```python
from build123d import *

# Parameters (mm, degrees)
F0_W     = 50.8
F0_H     = 25.4
F0_R     = 3
F1_DEPTH = 3.5
F2_DEPTH = 10.16
F3_SIZE  = 1.27
F4_SIZE  = 3.81
F0_R_2   = 1.75
F5_DEPTH = 2.54
F6_W     = 6.391182
F6_H     = 4.83196
F7_DEPTH = 31.592


with BuildPart() as f1:
    # F0 (on Top) → F1 (new body)
    with BuildSketch(Plane.XY):
        with Locations((2.701852, 34.358082)):
            Rectangle(F0_W, F0_H)
        Polygon((-19.831223, 38.395144), (-19.831223, 44.550914), (25.234927, 44.550914), (25.234927, 38.395144), (18.497852, 38.395144), (18.497852, 30.32102), (25.234927, 30.32102), (25.234927, 24.16525), (-19.831223, 24.16525), (-19.831223, 30.32102), (-13.094148, 30.32102), (-13.094148, 38.395144), align=None, mode=Mode.SUBTRACT)
        with Locations((-16.348148, 34.358082)):
            Circle(F0_R, mode=Mode.SUBTRACT)
        with Locations((21.751852, 34.358082)):
            Circle(F0_R, mode=Mode.SUBTRACT)
    extrude(amount=F1_DEPTH)

    # F0 (on Top) → F2 (join)
    with BuildSketch(Plane.XY):
        Polygon((25.234927, 44.550914), (-19.831223, 44.550914), (-19.831223, 38.395144), (-13.094148, 38.395144), (-13.094148, 30.32102), (-19.831223, 30.32102), (-19.831223, 24.16525), (25.234927, 24.16525), (25.234927, 30.32102), (18.497852, 30.32102), (18.497852, 38.395144), (25.234927, 38.395144), align=None)
    extrude(amount=F2_DEPTH)

    # F3
    f3_edges = [f1.edges().sort_by_distance(p)[0] for p in [
        (-22.698148, 34.358082, 3.5),
        (2.701852, 21.658082, 3.5),
        (2.701852, 47.058082, 3.5),
        (28.101852, 34.358082, 3.5),
        (-22.698148, 47.058082, 1.75),
        (-22.698148, 21.658082, 1.75),
        (28.101852, 21.658082, 1.75),
        (28.101852, 47.058082, 1.75),
    ]]
    chamfer(f3_edges, length=F3_SIZE)

    # F4
    f4_edges = [f1.edges().sort_by_distance(p)[0] for p in [
        (25.234927, 41.473029, 10.16),
        (2.701852, 44.550914, 10.16),
        (25.234927, 27.243135, 10.16),
        (2.701852, 24.16525, 10.16),
        (-19.831223, 41.473029, 10.16),
        (-19.831223, 27.243135, 10.16),
    ]]
    chamfer(f4_edges, length=F4_SIZE)

    # F0 (on Top) → F5 (join)
    with BuildSketch(Plane.XY):
        with Locations((21.751852, 34.358082)):
            Circle(F0_R)
        with Locations((21.751852, 34.358082)):
            Circle(F0_R_2, mode=Mode.SUBTRACT)
        with Locations((-16.348148, 34.358082)):
            Circle(F0_R)
        with Locations((-16.348148, 34.358082)):
            Circle(F0_R_2, mode=Mode.SUBTRACT)
    extrude(amount=F5_DEPTH)

    # F6 (on face) → F7 (cut, through all)
    with BuildSketch(Plane(origin=(-13.094148, 0, 0), x_dir=(0, -1, 0), z_dir=(-1, 0, 0))):
        with Locations((-34.358082, 6.83)):
            Rectangle(F6_W, F6_H)
    extrude(amount=-F7_DEPTH, mode=Mode.SUBTRACT)


solid = f1.part
```
Here's how the part is built. I have some questions about the finished solid (model axes, mm). A direction names the side the tool comes from. Coordinates: 2 decimals unless noted, no trailing zeros. Loops run counter-clockwise (first coordinate to the right, second up) from the corner with the lowest first, then second, coordinate; pieces in that order, holes last. Notation, with made-up numbers: (78, 79) - (92, 79) arc R6 ccw to (92, 88) - close; hole circle Ø2 at (74, -30). An arc over 180 degrees is marked (long way). Return JSON: item names as keys, results as strings. Group by question number.
Item 1: I need wall thicknesses on line 1 (Z direction, x = -13, y = 36.5); line 2 (Y direction, x = 22.5, z = 2.5); line 3 (Z direction, x = 20.5, y = 36.5). Which ranges of each line are inside material? Lowest first, please. Write a range as from..to.
Item 2: We'd pull the mould along Y, two halves only. Please class faces 6 (the face through (2.386, 26.097, 8.282)), 7 (the face through (22, 32, 2.54)), 8 (the face through (28.102, 34, 1)): +Y half, -Y half, draft (parallel to the pull), parting line (faces both ways), or undercut.
Item 3: If we section it at B-B on x = -6: Write out the boundary of the cut face in (y, z), and give its area (3 significant figures).
Item 4: If we section it at C-C on y = 23.5: Write out the boundary of the cut face in (x, z), and give its area (3 significant figures).
Item 5: On a 3-axis mill with a long thin cutter (end or side, diameter ignored), from which of +Z, -Z, +X, -X, +Y, -Y can I reach the whole of each face in a straight line? I mean faces 1 (the face through (2, 24.165, 5)), 2 (the face through (-13.094, 34, 4)), 3 (the face through (-19.831, 42, 5)), 4 (the face through (2, 37.554, 7)), 5 (the face through (25.235, 41, 5)). Say none if no direction works.
Item 6: Will these pins go through, and if not, where does the flat tip stop? P1, Ø4, axis at x = 2.5, z = 7, coming from the -Y side; P2, Ø3, axis at y = 43.5, z = 8.5, coming from the -X side; P3, Ø6, axis at x = -5.5, z = 7, coming from the +Y side.
Item 7: If we section it at A-A on z = 8.25: Write out the boundary of the cut face in (x, y).
Item 8: If we section it at D-D on z = 1.5: Write out the boundary of the cut face in (x, y).
Calculated:
{
 "1": {"line 1": "z = 0..4.41, 9.25..10.16", "line 2": "y = 21.93..32.78, 35.94..46.79", "line 3": "z = 0..2.54"},
 "2": {"face 6": "-Y half", "face 7": "undercut", "face 8": "draft"},
 "3": {"outline": "(21.66, 0) - (47.06, 0) - (47.06, 2.23) - (45.79, 3.5) - (44.55, 3.5) - (44.55, 6.35) - (40.74, 10.16) - (27.98, 10.16) - (24.17, 6.35) - (24.17, 3.5) - (22.93, 3.5) - (21.66, 2.23) - close; hole (31.16, 4.41) - (37.55, 4.41) - (37.55, 9.25) - (31.16, 9.25) - close", "area": "178 mm^2"},
 "4": {"outline": "(-22.7, 0) - (28.1, 0) - (28.1, 2.23) - (26.83, 3.5) - (-21.43, 3.5) - (-22.7, 2.23) - close", "area": "176 mm^2"},
 "5": {"face 1": "+Z, +X, -X, -Y", "face 2": "+Z, -X", "face 3": "+Z, -X, +Y, -Y", "face 4": "+X, -X", "face 5": "+Z, +X, +Y, -Y"},
 "6": {"P1": "stops at y = 24.17", "P2": "stops at x = -19.18", "P3": "stops at y = 44.55"},
 "7": {"outline": "(-17.93, 26.07) - (23.33, 26.07) - (23.33, 30.32) - (18.5, 30.32) - (18.5, 31.16) - (-13.09, 31.16) - (-13.09, 30.32) - (-17.93, 30.32) - close; (-17.93, 38.4) - (-13.09, 38.4) - (-13.09, 37.55) - (18.5, 37.55) - (18.5, 38.4) - (23.33, 38.4) - (23.33, 42.65) - (-17.93, 42.65) - close"},
 "8": {"outline": "(-22.7, 22.93) - (-21.43, 21.66) - (26.83, 21.66) - (28.1, 22.93) - (28.1, 45.79) - (26.83, 47.06) - (-21.43, 47.06) - (-22.7, 45.79) - close; hole circle Ø3.5 at (-16.35, 34.36); hole circle Ø3.5 at (21.75, 34.36)"}
}
